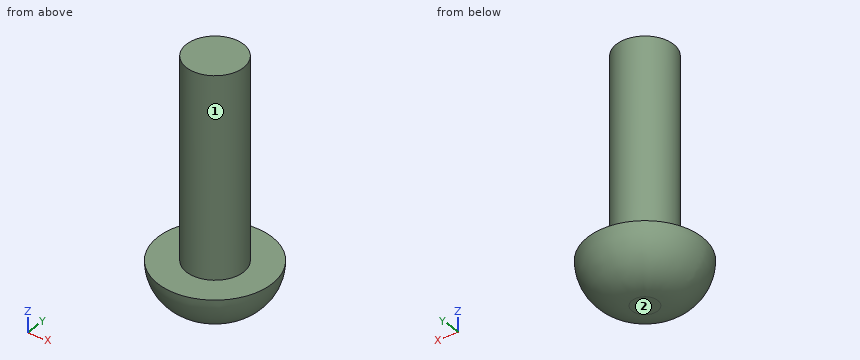
Autodesk Inventor part; units mm, degrees
ref_plane "YZ Plane" through (0, 0, 0) normal (1, 0, 0) x (0, 1, 0)
ref_plane "XZ Plane" through (0, 0, 0) normal (0, 1, 0) x (-1, 0, 0)
ref_plane "XY Plane" through (0, 0, 0) normal (0, 0, 1) x (1, 0, 0)
sketch "スケッチ1" plane through (0, 0, 0) normal (0, 0, 1) x (1, 0, 0)
  circle A0 centre (0, 0) radius 2
  dimension "d1" = 4
extrude "押し出し1" add sketch "スケッチ1" along normal blind 14
sketch "スケッチ2" plane through (0, 0, 0) normal (0, 0, -1) x (-1, 0, 0)
  circle A0 centre (0, 0) radius 2
  circle A1 centre (0, 0) radius 4
  dimension "d4" = 8
extrude "押し出し2" add sketch "スケッチ2" along normal blind 3.1 contours A0 | A1
fillet "フィレット1" radius 3.1 1 edges at (4, 0, -3.1)
thread "ねじ1"
properties part number "ネジ鍋m4,14" material "鋼、高強度、低合金"
CAD build for the part. Positions are in the model's coordinates, mm. Face numbers are marked on the shaded views. A direction names the side the tool comes from. Coordinates: 2 decimals unless noted, no trailing zeros. Loops run counter-clockwise (first coordinate to the right, second up) from the corner with the lowest first, then second, coordinate; pieces in that order, holes last. Notation, with made-up numbers: (64.25, 73.25) - (107.25, 73.25) arc R20 ccw to (107.25, 79.25) - close; hole circle Ø3 at (78.25, 80). An arc over 180 degrees is marked (long way). Use CSV: the item, a comma, the result in double quotes. Start each with the question number.
Q1. 3-axis set-ups, long thin cutter, end or side, ignore diameter. For the marked faces 1 and 2: which of +Z, -Z, +X, -X, +Y, -Y reach the whole face in a straight line?
Q2. Drop flat-ended pins along their axis: P1, Ø4, axis at y = -0.5, z = 7, coming from the -X side; P2, Ø4, axis at x = 0.5, z = 2.5, coming from the -Y side; P3, Ø3, axis at y = 1.5, z = -1, coming from the +X side. Give the stop position or say it passes through.
Q3. Probe probe 1 along Y at (x, z) = (0, 2.75); probe 2 along Z at (x, y) = (-2.75, -2); probe 3 along Z at (x, y) = (-3, -2.25). List the from-to ranges inside material, lowest first. Write a range as from..to.
Q4. Cut at A-A, the plane z = 10.25. List the corners of the cut face in (x, y).
Here are the results:
1,face 1,"+Z"
1,face 2,"-Z, +X, -X, +Y, -Y"
2,P1,"x = -2"
2,P2,"y = -2"
2,P3,"x = 3.99"
3,probe 1,"-2..2"
3,probe 2,"-1.83..0"
3,probe 3,"-1.22..0"
4,outline,"circle Ø4 at (0, 0)"
